Source: CAD feature listing. Evaluate the final solid. Frame: model axes, mm. Face numbers are marked on the shaded views. Round coordinates to 2 decimals unless told otherwise and drop trailing zeros. Write each loop counter-clockwise with the first axis right and the second up, starting at its lowest first coordinate (ties: lowest second). Pieces come first, ordered by that corner, then holes.
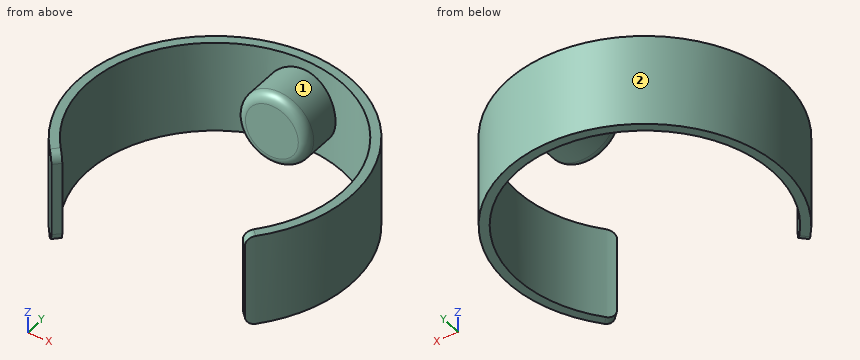
```python
from build123d import *

# Parameters (mm, degrees)
CYLINDER_W        = 15
CYLINDER_H        = 10
CYLINDER_ANGLE    = 270
CYLINDER001_W     = 14
CYLINDER001_H     = 10
CYLINDER001_ANGLE = 270
CYLINDER002_R     = 3.9
CYLINDER002_DEPTH = 5
FILLET_R          = 1
FILLET001_R       = 1


with BuildPart() as part:
    # Cylinder → Cylinder (revolve)
    with BuildSketch(Plane(origin=(0, 0, 0), x_dir=(0.707107, -0.707107, 0), z_dir=(-0.707107, -0.707107, 0))):
        with Locations((7.5, 5)):
            Rectangle(CYLINDER_W, CYLINDER_H)
    revolve(axis=Axis((0, 0, 0), (0, 0, 1)), revolution_arc=CYLINDER_ANGLE)

    # Cylinder001 → Cylinder001 (revolve, cut)
    with BuildSketch(Plane(origin=(0, 0, 0), x_dir=(0.707107, -0.707107, 0), z_dir=(-0.707107, -0.707107, 0))):
        with Locations((7, 5)):
            Rectangle(CYLINDER001_W, CYLINDER001_H)
    revolve(axis=Axis((0, 0, 0), (0, 0, 1)), revolution_arc=CYLINDER001_ANGLE, mode=Mode.SUBTRACT)

    # Cylinder002 → Cylinder002 (join)
    with BuildSketch(Plane(origin=(0, 14, 5), x_dir=(1, 0, 0), z_dir=(0, -1, 0))):
        Circle(CYLINDER002_R)
    extrude(amount=CYLINDER002_DEPTH)

    # Fillet
    fillet_edges = [part.edges().sort_by_distance(p)[0] for p in [
        (-3.9, 9, 5),
    ]]
    fillet(fillet_edges, radius=FILLET_R)

    # Fillet001
    fillet001_edges = [part.edges().sort_by_distance(p)[0] for p in [
        (-10.253048, -10.253048, 10),
        (-10.253048, -10.253048, 0),
        (10.253048, -10.253048, 0),
        (10.253048, -10.253048, 10),
    ]]
    fillet(fillet001_edges, radius=FILLET001_R)


solid = part.part
```
Q1. Pin query (flat end, axial travel): P1, Ø3, axis at x = 1, z = 8, coming from the -Y side; P2, Ø4, axis at y = -7.5, z = 2.5, coming from the -X side; P3, Ø4, axis at y = 10.5, z = 5.5, coming from the -X side. Return the tip coordinate at first contact, or that it passes through.
Q2. Section query A-A, the plane y = 0. Output: boundary loops of the cut face in (x, z), and give its area (3 significant figures).
Q3. Section query D-D, the plane y = 12. Output: boundary loops of the cut face in (x, z), and give its area (3 significant figures).
Q4. Mould query, pull axis X, two halves, no side actions, for the marked faces 1 and 2. Classes: pulls with the +X half, pulls with the -X half, needs draft (parallel to the pull), parting line crosses it, or undercut.
Q5. Line query: line 1 (X direction, y = 0, z = 5); line 2 (Y direction, x = 0, z = 4.75); line 3 (X direction, y = 13, z = 6.5). Output: solid intervals per line, ascending.
Q6. Section query C-C, the plane z = 5. Output: boundary loops of the cut face in (x, y).
Q7. Section query B-B, the plane x = 0. Output: boundary loops of the cut face in (y, z), and give its area (3 significant figures).
Filled in:
1. P1: stops at y = 9
1. P2: stops at x = -13.96
1. P3: stops at x = -12.36
2. outline: (-15, 0) - (-14, 0) - (-14, 10) - (-15, 10) - close; (14, 0) - (15, 0) - (15, 10) - (14, 10) - close
2. area: 20.0 mm2
3. outline: (-9, 0) - (-7.21, 0) - (-7.21, 10) - (-9, 10) - close; circle Ø7.8 at (0, 5); (7.21, 0) - (9, 0) - (9, 10) - (7.21, 10) - close
3. area: 83.6 mm2
4. face 1: undercut
4. face 2: parting line crosses it
5. line 1: x = -15 to -14, 14 to 15
5. line 2: y = 9 to 15
5. line 3: x = -7.48 to -5.2, -3.6 to 3.6, 5.2 to 7.48
6. outline: (-10.61, -10.61) - (-9.9, -9.9) arc R14 cw to (-3.9, 13.45) - (-3.9, 10) arc R1 ccw to (-2.9, 9) - (2.9, 9) arc R1 ccw to (3.9, 10) - (3.9, 13.45) arc R14 cw to (9.9, -9.9) - (10.61, -10.61) arc R15 ccw (long way) to start
7. outline: (9, 2.1) arc R1 ccw to (10, 1.1) - (14, 1.1) - (14, 0) - (15, 0) - (15, 10) - (14, 10) - (14, 8.9) - (10, 8.9) arc R1 ccw to (9, 7.9) - close
7. area: 48.6 mm2
